from build123d import *

# Parameters (mm, degrees)
SKETCH1_R           = 11.25
BOSS_EXTRUDE1_DEPTH = 12
SKETCH2_R           = 4.15
CUT_EXTRUDE1_DEPTH  = 15
SKETCH3_R           = 2.1
CUT_EXTRUDE2_DEPTH  = 5
SKETCH4_R           = 1.75
CUT_EXTRUDE3_DEPTH  = 18.5000001


with BuildPart() as part:
    # Sketch1 → Boss-Extrude1 (new body)
    with BuildSketch(Plane.XY):
        Circle(SKETCH1_R)
    extrude(amount=BOSS_EXTRUDE1_DEPTH)

    # Sketch2 → Cut-Extrude1 (cut)
    with BuildSketch(Plane.XY.offset(12)):
        Circle(SKETCH2_R)
    extrude(amount=-CUT_EXTRUDE1_DEPTH, mode=Mode.SUBTRACT)

    # Sketch3 → Cut-Extrude2 (cut)
    with BuildSketch(Plane(origin=(-11.25, 0, 0), x_dir=(0, 0, -1), z_dir=(1, 0, 0))):
        with Locations((-6, 0)):
            Circle(SKETCH3_R)
    cut_extrude2 = extrude(amount=CUT_EXTRUDE2_DEPTH, mode=Mode.SUBTRACT)

    # Sketch4 → Cut-Extrude3 (cut, through all)
    with BuildSketch(Plane.ZY.offset(6.25)):
        with Locations((6, 0)):
            Circle(SKETCH4_R)
    extrude(amount=-CUT_EXTRUDE3_DEPTH, mode=Mode.SUBTRACT)

    # Mirror1: Cut-Extrude2 across plane
    add(cut_extrude2.mirror(Plane(origin=(0, 0, 0), x_dir=(0, 0, 1), z_dir=(1, 0, 0))), mode=Mode.SUBTRACT)


solid = part.part
For this review, take the finished solid that the model builds, in its own axes (mm). A direction names the side the tool comes from. Round coordinates to 2 decimals unless told otherwise and drop trailing zeros. Write each loop counter-clockwise with the first axis right and the second up, starting at its lowest first coordinate (ties: lowest second). Pieces come first, ordered by that corner, then holes. Notation, with made-up numbers: (17.25, 21.25) - (73.25, 21.25) arc R20 ccw to (73.25, 33.25) - close; hole circle Ø11 at (1, 39.5). An arc over 180 degrees is marked (long way). Write item = value, one per line. Start each with the question number.
1. For faces 1 (the face through (8.78, 0.09, 8.1)), 2 (the face through (-8.79, 0.09, 8.1)), 3 (the face through (-5.024, 0.526, 7.669)), list the 3-axis set-ups (+Z, -Z, +X, -X, +Y, -Y) from which the entire face can be reached by the end or side of a thin tool; tool diameter is ignored.
2. Draft analysis for pull direction Y (two halves, no side actions). For faces 4 (the face through (5, 0, 12)), 5 (the face through (10.39, -4.31, 5.92)), 6 (the face through (4.989, 0.526, 7.669)), state which applies: released by +Y, released by -Y, zero draft, split by the parting line, or undercut.
3. Consider section C-C on z = 7.25. State the section outline as (x, y) points.
4. Wall thickness on L1, parallel to Y at x = 0, z = 4.5; L2, parallel to Y at x = -4.3, z = 6; L3, parallel to X at y = -1.75, z = 3: over which ranges is each line inside the solid? List them lowest first.
5. Consider section B-B on x = 0. State the section outline as (y, z) points.
6. For pin 1 Ø8 at (x, y) = (-7.5, 0.5) entering from -Z; pin 2 Ø2 at (y, z) = (3.5, 4.5) entering from -X; pin 3 Ø2 at (y, z) = (-1, 5) entering from -X, all flat-tipped, find the tip position at first contact; note any pin that passes through.
7. Consider section A-A on y = 0. State the section outline as (x, z) points, plus the area to 3 significant figures.
8. Consider section D-D on x = -9. State the section outline as (y, z) points, plus the area to 3 significant figures.
Evaluation:
q1.face_1 = +X
q1.face_2 = -X
q1.face_3 = +X, -X
q2.face_4 = zero draft
q2.face_5 = split by the parting line
q2.face_6 = undercut
q3.outline = (-11.12, -1.69) arc R11.25 ccw to (11.12, -1.69) - (6.25, -1.69) - (6.25, -1.22) - (3.97, -1.22) arc R4.15 cw to (-3.97, -1.22) - (-6.25, -1.22) - (-6.25, -1.69) - close; (-11.12, 1.69) - (-6.25, 1.69) - (-6.25, 1.22) - (-3.97, 1.22) arc R4.15 cw to (3.97, 1.22) - (6.25, 1.22) - (6.25, 1.69) - (11.12, 1.69) arc R11.25 ccw to start
q4.L1 = -11.25 to -4.15, 4.15 to 11.25
q4.L2 = -10.4 to -1.75, 1.75 to 10.4
q4.L3 = -11.11 to -3.76, 3.76 to 11.11
q5.outline = (-11.25, 0) - (-4.15, 0) - (-4.15, 12) - (-11.25, 12) - close; (4.15, 0) - (11.25, 0) - (11.25, 12) - (4.15, 12) - close
q6.pin_1 = 0
q6.pin_2 = -10.97
q6.pin_3 = -11.23
q7.outline = (-11.25, 0) - (-4.15, 0) - (-4.15, 4.25) - (-6.25, 4.25) - (-6.25, 3.9) - (-11.25, 3.9) - close; (-11.25, 8.1) - (-6.25, 8.1) - (-6.25, 7.75) - (-4.15, 7.75) - (-4.15, 12) - (-11.25, 12) - close; (4.15, 0) - (11.25, 0) - (11.25, 3.9) - (6.25, 3.9) - (6.25, 4.25) - (4.15, 4.25) - close; (4.15, 7.75) - (6.25, 7.75) - (6.25, 8.1) - (11.25, 8.1) - (11.25, 12) - (4.15, 12) - close
q7.area = 114 mm2
q8.outline = (-6.75, 0) - (6.75, 0) - (6.75, 12) - (-6.75, 12) - close; hole circle Ø4.2 at (0, 6)
q8.area = 148 mm2
